from build123d import *

# Parameters (mm, degrees)
SKETCH1_R           = 175
SKETCH1_R_2         = 125
SKETCH1_R_3         = 6.1
BOSS_EXTRUDE1_DEPTH = 5


with BuildPart() as part:
    # Sketch1 → Boss-Extrude1 (new, symmetric)
    with BuildSketch(Plane(origin=(0, 0, 0), x_dir=(1, 0, 0), z_dir=(0, 1, 0))):
        with Locations(Location((0, 0, 0), (0, 0, 270))):
            Circle(SKETCH1_R)
        with Locations(Location((0, 0, 0), (0, 0, 270))):
            Circle(SKETCH1_R_2, mode=Mode.SUBTRACT)
        with Locations(Location((0, 150, 0), (0, 0, 270))):
            Circle(SKETCH1_R_3, mode=Mode.SUBTRACT)
        with Locations(Location((57.402514855, 138.581929877, 0), (0, 0, 270))):
            Circle(SKETCH1_R_3, mode=Mode.SUBTRACT)
        with Locations(Location((106.066017178, 106.066017178, 0), (0, 0, 270))):
            Circle(SKETCH1_R_3, mode=Mode.SUBTRACT)
        with Locations(Location((138.581929877, 57.402514855, 0), (0, 0, 270))):
            Circle(SKETCH1_R_3, mode=Mode.SUBTRACT)
        with Locations(Location((150, 0, 0), (0, 0, 270))):
            Circle(SKETCH1_R_3, mode=Mode.SUBTRACT)
        with Locations(Location((138.581929877, -57.402514855, 0), (0, 0, 270))):
            Circle(SKETCH1_R_3, mode=Mode.SUBTRACT)
        with Locations(Location((106.066017178, -106.066017178, 0), (0, 0, 270))):
            Circle(SKETCH1_R_3, mode=Mode.SUBTRACT)
        with Locations(Location((57.402514855, -138.581929877, 0), (0, 0, 270))):
            Circle(SKETCH1_R_3, mode=Mode.SUBTRACT)
        with Locations(Location((0, -150, 0), (0, 0, 270))):
            Circle(SKETCH1_R_3, mode=Mode.SUBTRACT)
        with Locations(Location((-57.402514855, -138.581929877, 0), (0, 0, 270))):
            Circle(SKETCH1_R_3, mode=Mode.SUBTRACT)
        with Locations(Location((-106.066017178, -106.066017178, 0), (0, 0, 270))):
            Circle(SKETCH1_R_3, mode=Mode.SUBTRACT)
        with Locations(Location((-138.581929877, -57.402514855, 0), (0, 0, 270))):
            Circle(SKETCH1_R_3, mode=Mode.SUBTRACT)
        with Locations(Location((-150, 0, 0), (0, 0, 270))):
            Circle(SKETCH1_R_3, mode=Mode.SUBTRACT)
        with Locations(Location((-138.581929877, 57.402514855, 0), (0, 0, 270))):
            Circle(SKETCH1_R_3, mode=Mode.SUBTRACT)
        with Locations(Location((-106.066017178, 106.066017178, 0), (0, 0, 270))):
            Circle(SKETCH1_R_3, mode=Mode.SUBTRACT)
        with Locations(Location((-57.402514855, 138.581929877, 0), (0, 0, 270))):
            Circle(SKETCH1_R_3, mode=Mode.SUBTRACT)
    extrude(amount=BOSS_EXTRUDE1_DEPTH, both=True)


solid = part.part
Model file for the job. Use its own axes, mm. Give positions to 0.01 mm unless a question says otherwise; leave off trailing zeros. Write each loop counter-clockwise with the first axis right and the second up, starting at its lowest first coordinate (ties: lowest second). Pieces come first, ordered by that corner, then holes. Notation, with made-up numbers: M 71,-2 L 84,-2 A20 cw 84,28 Z; hole C 74,67.25 d2. An arc over 180 degrees is marked long. One line per item, written item: value. Start each with the question number.
Q1. Saw through at C-C, the plane y = -0.25. State how many separate pieces and enclosed holes the cut face has, plus the area to 3 significant figures.
Q2. Drop flat-ended pins along their axis: pin 1 Ø7.5 at (x, z) = (-138.58, -57.4) entering from +Y; pin 2 Ø6 at (x, y) = (89, -1) entering from +Z; pin 3 Ø2 at (x, y) = (-71.5, -4) entering from -Z; pin 4 Ø5 at (x, y) = (-109, -1) entering from +Z. Give the stop position or say it passes through.
Q3. Saw through at A-A, the plane z = 0. Write the cut outline in (x, y), plus the area to 3 significant figures.
Q4. Saw through at B-B, the plane x = 0. Write the cut outline in (y, z), plus the area to 3 significant figures.
Q5. Saw through at D-D, the plane x = 121. Write the cut outline in (y, z).
Q6. Two-plate mould, pull along X, no slides. Class faces 1 (the flat face through (117, 5, -53)), 2 (the cylindrical face through (173.51, 0.07, -22.78)), 3 (the cylindrical face through (100.11, -0.07, -107.39)): +X half, -X half, draft (parallel to the pull), parting line (faces both ways), or undercut.
Q7. Probe probe 1 along X at (y, z) = (0.5, 0); probe 2 along Z at (x, y) = (-104.5, -3); probe 3 along Z at (x, y) = (60, -1.25). List the from-to ranges inside material, lowest first. Write a range as [from, to].
Output values:
1. separate pieces: 1
1. enclosed holes: 17
1. area: 45,300 mm²
2. pin 1: passes through
2. pin 2: stops at z = 152.41
2. pin 3: stops at z = -160.17
2. pin 4: stops at z = 138.86
3. outline: M -175,-5 L -156.1,-5 L -156.1,5 L -175,5 Z; M -143.9,-5 L -125,-5 L -125,5 L -143.9,5 Z; M 125,-5 L 143.9,-5 L 143.9,5 L 125,5 Z; M 156.1,-5 L 175,-5 L 175,5 L 156.1,5 Z
3. area: 756 mm²
4. outline: M -5,-175 L 5,-175 L 5,-156.1 L -5,-156.1 Z; M -5,-143.9 L 5,-143.9 L 5,-125 L -5,-125 Z; M -5,125 L 5,125 L 5,143.9 L -5,143.9 Z; M -5,156.1 L 5,156.1 L 5,175 L -5,175 Z
4. area: 756 mm²
5. outline: M -5,-126.43 L 5,-126.43 L 5,-31.37 L -5,-31.37 Z; M -5,31.37 L 5,31.37 L 5,126.43 L -5,126.43 Z
6. face 1: draft
6. face 2: parting line
6. face 3: undercut
7. probe 1: x = [-175, -156.1], [-143.9, -125], [125, 143.9], [156.1, 175]
7. probe 2: z = [-140.37, -111.96], [-100.17, -68.59], [68.59, 100.17], [111.96, 140.37]
7. probe 3: z = [-164.39, -144.1], [-133.06, -109.66], [109.66, 133.06], [144.1, 164.39]
